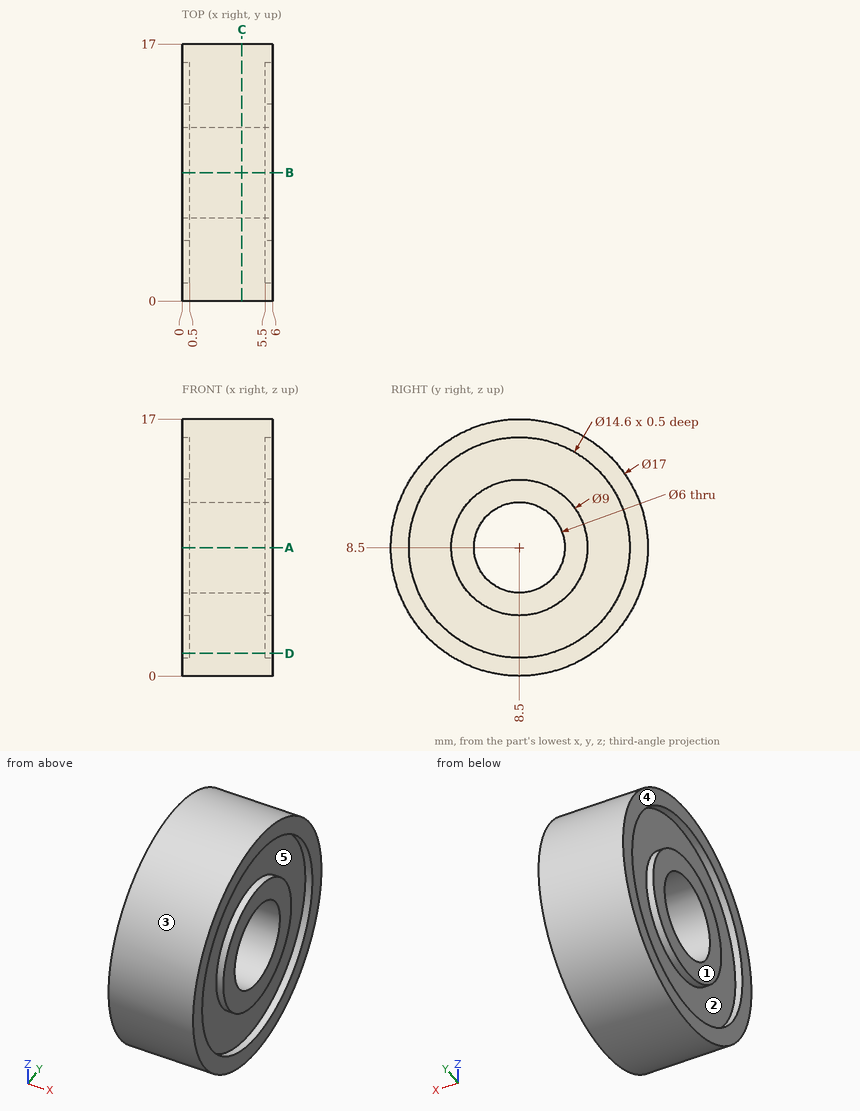
Source: three-view drawing plus pictorial views. Frame: mm from the lowest corner of the part. A direction names the side the tool comes from. Give positions to 0.01 mm unless a question says otherwise; leave off trailing zeros. Write each loop counter-clockwise with the first axis right and the second up, starting at its lowest first coordinate (ties: lowest second). Pieces come first, ordered by that corner, then holes. Notation, with made-up numbers: (-15.5, 54.25) - (28.5, 54.25) arc R27 ccw to (28.5, 89.25) - close; hole circle Ø2 at (24.25, 22). An arc over 180 degrees is marked (long way). Write item = value, one per line. Start each with the question number.
1. Mould query, pull axis Z, two halves, no side actions, for the marked faces 1, 2 and 3. Classes: released by +Z, released by -Z, zero draft, split by the parting line, or undercut.
2. Section query C-C, the plane x = 3.95. Output: boundary loops of the cut face in (y, z), then the cut area to 3 significant figures.
3. Section query A-A, the plane z = 8.5. Output: boundary loops of the cut face in (x, y).
4. Section query D-D, the plane z = 1.5. Output: boundary loops of the cut face in (x, y), then the cut area to 3 significant figures.
5. Ray query, L1, parallel to Y at x = 5.7, z = 8.5; L2, parallel to Y at x = 2.45, z = 8.5; L3, parallel to X at y = 13.75, z = 10.75. Return the intervals inside material, ascending.
6. Access query for the marked faces 4 and 5. Directions: +Z, -Z, +X, -X, +Y, -Y. A direction counts if a zero-diameter tool reaches every point of the face in a straight line with its end or side. Return the directions, or none.
7. First-contact query: pin 1 Ø5 at (y, z) = (9, 6) entering from -X; pin 2 Ø1 at (x, y) = (3, 11.5) entering from +Z; pin 3 Ø2 at (x, z) = (3.5, 4.5) entering from +Y; pin 4 Ø1.5 at (x, z) = (2.5, 4) entering from -Y. Flat tips, straight axial feed; report the tip coordinate or a pass-through.
Check sheet entries:
q1.face_1 = zero draft
q1.face_2 = undercut
q1.face_3 = split by the parting line
q2.outline = circle Ø17 at (8.5, 8.5); hole circle Ø6 at (8.5, 8.5)
q2.area = 199 mm2
q3.outline = (0, 0) - (6, 0) - (6, 1.2) - (5.5, 1.2) - (5.5, 4) - (6, 4) - (6, 5.5) - (0, 5.5) - (0, 4) - (0.5, 4) - (0.5, 1.2) - (0, 1.2) - close; (0, 11.5) - (6, 11.5) - (6, 13) - (5.5, 13) - (5.5, 15.8) - (6, 15.8) - (6, 17) - (0, 17) - (0, 15.8) - (0.5, 15.8) - (0.5, 13) - (0, 13) - close
q4.outline = (0, 3.68) - (6, 3.68) - (6, 6.43) - (5.5, 6.43) - (5.5, 10.57) - (6, 10.57) - (6, 13.32) - (0, 13.32) - (0, 10.57) - (0.5, 10.57) - (0.5, 6.43) - (0, 6.43) - close
q4.area = 53.7 mm2
q5.L1 = 0 to 1.2, 4 to 5.5, 11.5 to 13, 15.8 to 17
q5.L2 = 0 to 5.5, 11.5 to 17
q5.L3 = 0.5 to 5.5
q6.face_4 = +Z, -Z, -X, +Y, -Y
q6.face_5 = +X
q7.pin_1 = 0
q7.pin_2 = 16.62
q7.pin_3 = 16.45
q7.pin_4 = 0.87
